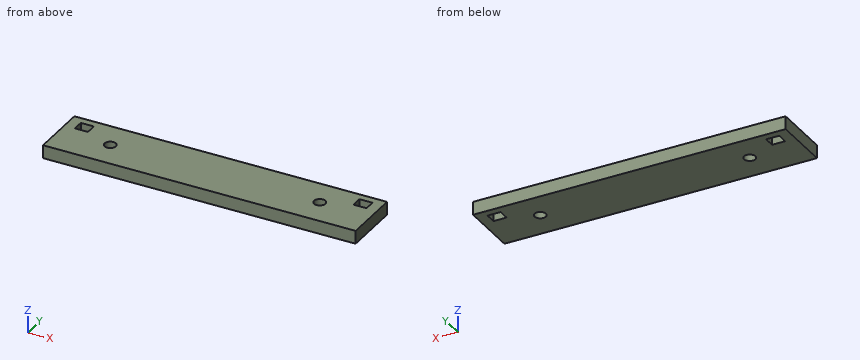
```python
from build123d import *

# Parameters (mm, degrees)
SKETCH1_W           = 37.8968
SKETCH1_H           = 6.985
SKETCH1_R           = 0.6858
SKETCH1_W_2         = 1.5875
SKETCH1_H_2         = 1.3208
BOSS_EXTRUDE1_DEPTH = 1.5875


with BuildPart() as part:
    # Sketch1 → Boss-Extrude1 (new body)
    with BuildSketch(Plane.XY):
        Rectangle(SKETCH1_W, SKETCH1_H)
        with Locations((-12.7, 0)):
            Circle(SKETCH1_R, mode=Mode.SUBTRACT)
        with Locations(Location((12.7, 0, 0), (0, 0, 180))):
            Circle(SKETCH1_R, mode=Mode.SUBTRACT)
        with Locations((-16.88465, 1.9304)):
            Rectangle(SKETCH1_W_2, SKETCH1_H_2, mode=Mode.SUBTRACT)
        with Locations((16.88465, 1.9304)):
            Rectangle(SKETCH1_W_2, SKETCH1_H_2, mode=Mode.SUBTRACT)
    extrude(amount=BOSS_EXTRUDE1_DEPTH)


solid = part.part
```
Source: CAD feature listing. Evaluate the final solid. Frame: model axes, mm. Give positions to 0.01 mm unless a question says otherwise; leave off trailing zeros. Write each loop counter-clockwise with the first axis right and the second up, starting at its lowest first coordinate (ties: lowest second). Pieces come first, ordered by that corner, then holes. Notation, with made-up numbers: (14, 65) - (18, 65) arc R25 ccw to (18, 77) - close; hole circle Ø6 at (30.5, -20.5). An arc over 180 degrees is marked (long way). One line per item, written item: value. Start each with the question number.
Q1. Section query C-C, the plane z = 1.15. Return the cut outline in (x, y).
Q2. First-contact query: pin 1 Ø1.1 at (x, y) = (-12.7, 0) entering from -Z. Flat tip, straight axial feed; report the tip coordinate or a pass-through.
Q3. Material intervals for probe 1 along X at (y, z) = (1.75, 0.6); probe 2 along Y at (x, z) = (12.7, 0.55); probe 3 along X at (y, z) = (0.5, 1.3), sorted ascending. Write a range as from..to.
Q4. Section query A-A, the plane y = 0. Return the cut outline in (x, z).
Q5. Section query D-D, the plane x = 12.5. Return the cut outline in (y, z).
Q6. Section query B-B, the plane x = -12.7. Return the cut outline in (y, z), then the cut area to 3 significant figures.
Answer:
1. outline: (-18.95, -3.49) - (18.95, -3.49) - (18.95, 3.49) - (-18.95, 3.49) - close; hole (-17.68, 1.27) - (-16.09, 1.27) - (-16.09, 2.59) - (-17.68, 2.59) - close; hole circle Ø1.37 at (-12.7, 0); hole circle Ø1.37 at (12.7, 0); hole (16.09, 1.27) - (17.68, 1.27) - (17.68, 2.59) - (16.09, 2.59) - close
2. pin 1: passes through
3. probe 1: x = -18.95..-17.68, -16.09..16.09, 17.68..18.95
3. probe 2: y = -3.49..-0.69, 0.69..3.49
3. probe 3: x = -18.95..-13.17, -12.23..12.23, 13.17..18.95
4. outline: (-18.95, 0) - (-13.39, 0) - (-13.39, 1.59) - (-18.95, 1.59) - close; (-12.01, 0) - (12.01, 0) - (12.01, 1.59) - (-12.01, 1.59) - close; (13.39, 0) - (18.95, 0) - (18.95, 1.59) - (13.39, 1.59) - close
5. outline: (-3.49, 0) - (-0.66, 0) - (-0.66, 1.59) - (-3.49, 1.59) - close; (0.66, 0) - (3.49, 0) - (3.49, 1.59) - (0.66, 1.59) - close
6. outline: (-3.49, 0) - (-0.69, 0) - (-0.69, 1.59) - (-3.49, 1.59) - close; (0.69, 0) - (3.49, 0) - (3.49, 1.59) - (0.69, 1.59) - close
6. area: 8.91 mm2
